Answer from the drawing. Dimensions are ordinates in mm from the lowest x, y and z of the part. Coordinates: 2 decimals unless noted, no trailing zeros. Loops run counter-clockwise (first coordinate to the right, second up) from the corner with the lowest first, then second, coordinate; pieces in that order, holes last. Notation, with made-up numbers: M 76,15.5 L 110,15.5 A22 ccw 110,43.5 Z; hole C -30.5,10.25 d10. An arc over 180 degrees is marked long. One line per item, written item: value. Start each with the question number.
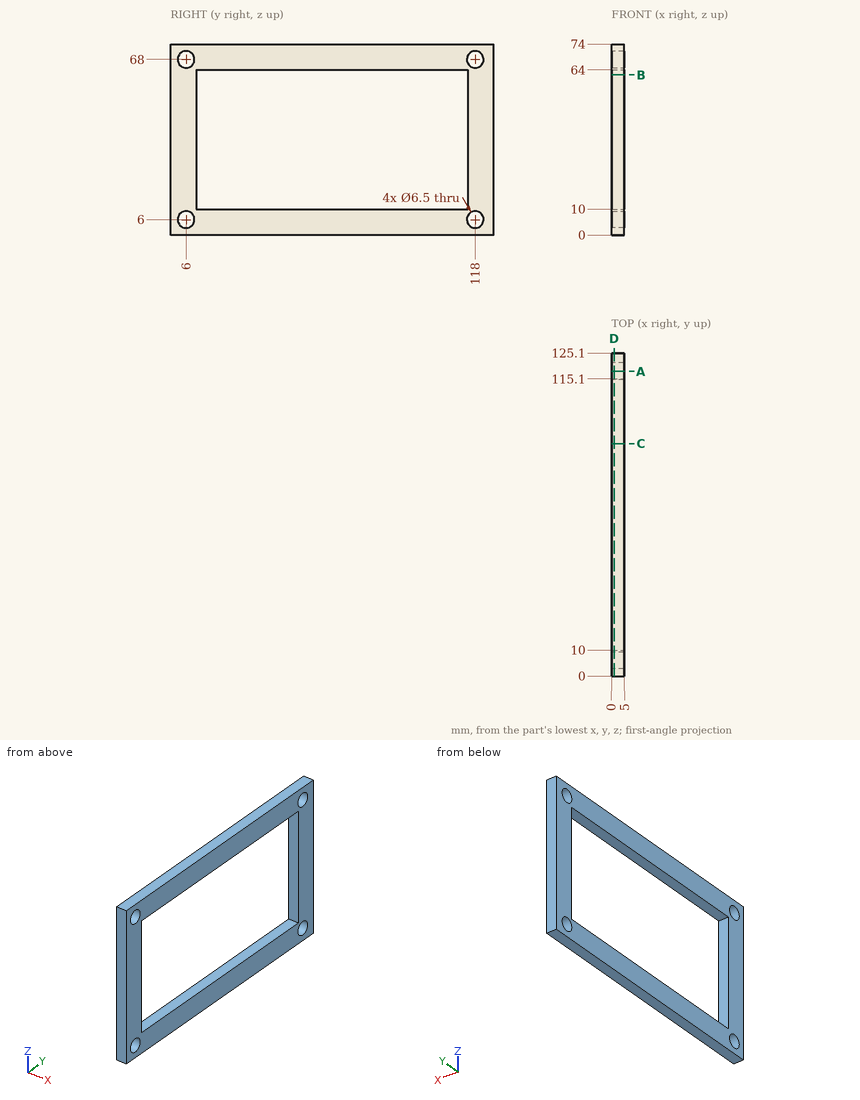
1) Section C-C (y = 90) is taken. Determine the outline of the cut face in (x, z), then the cut area to 3 significant figures.
2) Section B-B (z = 62) is taken. Determine the outline of the cut face in (x, y).
3) Consider line 1 along Y through (x, z) = (2.1, 68); line 2 along Y through (x, z) = (3.8, 51.5); line 3 along Z through (x, y) = (2.35, 13). Determine where each line is inside the solid, lowest interval first.
4) Section A-A (y = 118) is taken. Determine the outline of the cut face in (x, z), then the cut area to 3 significant figures.
5) A flat-ended cylindrical pin translates along its axis: pin 1 (6 mm diameter, centred on y = 118, z = 6, fed in from +X). Find the tip coordinate at first contact, or state that the pin passes through.
6) Section D-D (x = 1.05) is taken. Determine the outline of the cut face in (y, z), then the cut area to 3 significant figures.
Results found:
1. outline: M 0,0 L 5,0 L 5,10 L 0,10 Z; M 0,64 L 5,64 L 5,74 L 0,74 Z
1. area: 100 mm²
2. outline: M 0,0 L 5,0 L 5,10 L 0,10 Z; M 0,115.1 L 5,115.1 L 5,125.1 L 0,125.1 Z
3. line 1: y = 0 to 2.75, 9.25 to 114.75, 121.25 to 125.1
3. line 2: y = 0 to 10, 115.1 to 125.1
3. line 3: z = 0 to 10, 64 to 74
4. outline: M 0,0 L 5,0 L 5,2.75 L 0,2.75 Z; M 0,9.25 L 5,9.25 L 5,64.75 L 0,64.75 Z; M 0,71.25 L 5,71.25 L 5,74 L 0,74 Z
4. area: 305 mm²
5. pin 1: passes through
6. outline: M 0,0 L 125.1,0 L 125.1,74 L 0,74 Z; hole C 6,6 d6.5; hole C 6,68 d6.5; hole M 10,10 L 115.1,10 L 115.1,64 L 10,64 Z; hole C 118,6 d6.5; hole C 118,68 d6.5
6. area: 3,450 mm²
